Input: part model. Units: mm. Frame: model coordinates. A direction names the side the tool comes from. Round coordinates to 2 decimals unless told otherwise and drop trailing zeros. Loops run counter-clockwise (first coordinate to the right, second up) from the corner with the lowest first, then second, coordinate; pieces in that order, holes last.
(1) Cut plane B-B, the plane x = -5. Output: boundary loops of the cut face in (y, z), and give its area (3 significant figures).
(2) Access query for faces 4 (the face through (0, 0, 3)), 5 (the face through (-9.462, -1.724, 1.014)), 6 (the face through (-11, 2, 2)). Directions: +Z, -Z, +X, -X, +Y, -Y. A direction counts if a zero-diameter tool reaches every point of the face in a straight line with its end or side. Return the directions, or none.
(3) Line query: line 1 (X direction, y = -3.5, z = 0.25); line 2 (Y direction, x = -8.5, z = -4); line 3 (X direction, y = -0.5, z = 0). Output: solid intervals per line, ascending.
(4) First-contact query: pin 1 Ø1.5 at (x, y) = (1.5, 0.5) entering from -Z; pin 2 Ø4 at (x, z) = (-4, 1) entering from -Y; pin 3 Ø0.7 at (x, y) = (-9, 0.5) entering from +Z. Flat tips, straight axial feed; report the tip coordinate or a pass-through.
(5) Draft query along Y for faces 1 (the face through (-8.77, -1.08, 4.88)), 2 (the face through (7, 0, 0)), 3 (the face through (-9.46, 1.74, 0.99)). Return one class per face: released by +Y, released by -Y, zero draft, split by the parting line, or undercut.
(6) Cut plane A-A, the plane y = 0. Output: boundary loops of the cut face in (x, z).
from build123d import *

# Parameters (mm, degrees)
SKETCH2_R           = 3
BOSS_EXTRUDE1_DEPTH = 14
CHAMFER1_SIZE       = 0.75
CUT_EXTRUDE1_DEPTH  = 3.12


with BuildPart() as part:
    # Sketch2 → Boss-Extrude1 (new body)
    with BuildSketch(Plane(origin=(7, 0, 0), x_dir=(0, 0, -1), z_dir=(1, 0, 0))):
        Circle(SKETCH2_R)
    extrude(amount=-BOSS_EXTRUDE1_DEPTH)

    # Chamfer1
    chamfer1_edges = [part.edges().sort_by_distance(p)[0] for p in [
        (7, 0, 3),
    ]]
    chamfer(chamfer1_edges, length=CHAMFER1_SIZE)

    # Sketch6 → Revolve1 (revolve)
    with BuildSketch(Plane.XY):
        Polygon((-10.5, 5), (-11, 4.5), (-11, 0), (-7, 0), (-7, 5), align=None)
    revolve(axis=Axis((-7, 0, 0), (-1, 0, 0)))

    # Sketch4 → Cut-Extrude1 (cut)
    with BuildSketch(Plane(origin=(-11, 0, 0), x_dir=(0, 0, -1), z_dir=(1, 0, 0))):
        Polygon((0, 2.309401077), (-2, 1.154700538), (-2, -1.154700538), (0, -2.309401077), (2, -1.154700538), (2, 1.154700538), align=None)
    extrude(amount=CUT_EXTRUDE1_DEPTH, mode=Mode.SUBTRACT)

    # Cut-Extrude2 cone 1 section (through the dimple's axis) → Cut-Extrude2 (revolve, cut)
    with BuildSketch(Plane(origin=(-11, 0, 0), x_dir=(0, 0, 1), z_dir=(0, 1, 0))):
        Polygon((0, 0), (2.309401077, 0), (0, 2.309401077), align=None)
    revolve(axis=Axis((-11, 0, 0), (1, 0, 0)), mode=Mode.SUBTRACT)


solid = part.part
Reported:
1. outline: circle Ø6 at (0, 0)
1. area: 28.3 mm2
2. face 4: +X
2. face 5: -X
2. face 6: +Z, -Z, -X, +Y, -Y
3. line 1: x = -11 to -7
3. line 2: y = -3 to 3
3. line 3: x = -7.88 to 7
4. pin 1: stops at z = -3
4. pin 2: stops at y = -3
4. pin 3: stops at z = 5
5. face 1: split by the parting line
5. face 2: zero draft
5. face 3: undercut
6. outline: (-11, -4.5) - (-10.5, -5) - (-7, -5) - (-7, -3) - (6.25, -3) - (7, -2.25) - (7, 2.25) - (6.25, 3) - (-7, 3) - (-7, 5) - (-10.5, 5) - (-11, 4.5) - (-11, 2.31) - (-10.69, 2) - (-7.88, 2) - (-7.88, -2) - (-10.69, -2) - (-11, -2.31) - close
